```python
from build123d import *

# Parameters (mm, degrees)
F1_DEPTH = 25.4


with BuildPart() as f1:
    # F0 (on Front) → F1 (new body)
    with BuildSketch(Plane.XZ):
        with BuildLine():
            Line((-514.35, 714.375), (-522.739805, 714.375))
            ThreePointArc((-522.739805, 714.375), (-538.640068, 709.542625), (-549.162481, 696.679926))
            Line((-549.162481, 696.679926), (-578.52656, 625.367164))
            ThreePointArc((-578.52656, 625.367164), (-585.141661, 603.436284), (-587.375, 580.638581))
            Line((-587.375, 580.638581), (-587.375, 577.85))
            Line((-587.375, 577.85), (-587.375, 133.35))
            Line((-587.375, 133.35), (-587.375, 130.561419))
            ThreePointArc((-587.375, 130.561419), (-585.141661, 107.763716), (-578.52656, 85.832836))
            Line((-578.52656, 85.832836), (-549.162481, 14.520074))
            ThreePointArc((-549.162481, 14.520074), (-538.640068, 1.657375), (-522.739805, -3.175))
            Line((-522.739805, -3.175), (-514.35, -3.175))
            Line((-514.35, -3.175), (-69.85, -3.175))
            Line((-69.85, -3.175), (-61.460195, -3.175))
            ThreePointArc((-61.460195, -3.175), (-45.559932, 1.657375), (-35.037519, 14.520074))
            Line((-35.037519, 14.520074), (-5.67344, 85.832836))
            ThreePointArc((-5.67344, 85.832836), (0.941661, 107.763716), (3.175, 130.561419))
            Line((3.175, 130.561419), (3.175, 133.35))
            Line((3.175, 133.35), (3.175, 577.85))
            Line((3.175, 577.85), (3.175, 580.638581))
            ThreePointArc((3.175, 580.638581), (0.941661, 603.436284), (-5.67344, 625.367164))
            Line((-5.67344, 625.367164), (-35.037519, 696.679926))
            ThreePointArc((-35.037519, 696.679926), (-45.559932, 709.542625), (-61.460195, 714.375))
            Line((-61.460195, 714.375), (-69.85, 714.375))
            Line((-69.85, 714.375), (-514.35, 714.375))
        make_face()
        with BuildLine():
            Line((-522.739805, 711.2), (-514.35, 711.2))
            Line((-514.35, 711.2), (-69.85, 711.2))
            Line((-69.85, 711.2), (-61.460195, 711.2))
            ThreePointArc((-61.460195, 711.2), (-47.326628, 706.904556), (-37.973371, 695.471045))
            Line((-37.973371, 695.471045), (-8.609293, 624.158284))
            ThreePointArc((-8.609293, 624.158284), (-2.172979, 602.82013), (0, 580.638581))
            Line((0, 580.638581), (0, 577.85))
            Line((0, 577.85), (0, 133.35))
            Line((0, 133.35), (0, 130.561419))
            ThreePointArc((0, 130.561419), (-2.172979, 108.37987), (-8.609293, 87.041716))
            Line((-8.609293, 87.041716), (-37.973371, 15.728955))
            ThreePointArc((-37.973371, 15.728955), (-47.326628, 4.295444), (-61.460195, 0))
            Line((-61.460195, 0), (-69.85, 0))
            Line((-69.85, 0), (-514.35, 0))
            Line((-514.35, 0), (-522.739805, 0))
            ThreePointArc((-522.739805, 0), (-536.873372, 4.295444), (-546.226629, 15.728955))
            Line((-546.226629, 15.728955), (-575.590707, 87.041716))
            ThreePointArc((-575.590707, 87.041716), (-582.027021, 108.37987), (-584.2, 130.561419))
            Line((-584.2, 130.561419), (-584.2, 133.35))
            Line((-584.2, 133.35), (-584.2, 577.85))
            Line((-584.2, 577.85), (-584.2, 580.638581))
            ThreePointArc((-584.2, 580.638581), (-582.027021, 602.82013), (-575.590707, 624.158284))
            Line((-575.590707, 624.158284), (-546.226629, 695.471045))
            ThreePointArc((-546.226629, 695.471045), (-536.873372, 706.904556), (-522.739805, 711.2))
        make_face(mode=Mode.SUBTRACT)
    extrude(amount=F1_DEPTH)


solid = f1.part
```
Work out the finished part from the listing and answer in its coordinate system (mm). A direction names the side the tool comes from. Round coordinates to 2 decimals unless told otherwise and drop trailing zeros. Write each loop counter-clockwise with the first axis right and the second up, starting at its lowest first coordinate (ties: lowest second). Pieces come first, ordered by that corner, then holes. Notation, with made-up numbers: (-17, -37) -> (32, -37) arc R25 ccw to (32, -10) -> close; hole circle Ø4 at (-4.5, 39.25). An arc over 180 degrees is marked (long way). Write each question's results on one line, items separated by ' | '.
Q1. Section B-B, the plane z = 355 is taken. Write down the section's boundary in (x, y) (3 decimals).
Data:
outline: (-587.375, -25.4) -> (-584.2, -25.4) -> (-584.2, 0) -> (-587.375, 0) -> close; (0, -25.4) -> (3.175, -25.4) -> (3.175, 0) -> (0, 0) -> close
Q2. Which of the six approach directions +Z, -Z, +X, -X, +Y, -Y give full straight-line access (tool end or side, diameter ignored) to faces 5 (the flat face through (-23.497, -12.522, 660.314)), 6 (the flat face through (-587.375, -13, 359))?
Data:
face 5: +Y, -Y | face 6: +Z, -Z, -X, +Y, -Y
Q3. Section A-A, the plane x = -295 is taken. Write down the section's boundary in (y, z) (3 decimals).
Data:
outline: (-25.4, -3.175) -> (0, -3.175) -> (0, 0) -> (-25.4, 0) -> close; (-25.4, 711.2) -> (0, 711.2) -> (0, 714.375) -> (-25.4, 714.375) -> close
Q4. Straight lines are drawn through the part: line 1 along Z through (x, y) = (-205, -22.75) (3 decimals); line 2 along X through (y, z) = (-10.5, 560.5) (3 decimals); line 3 along X through (y, z) = (-16.75, 70). For each, find the intervals that lie inside material, in ascending order. Write a range as [from, to].
Data:
line 1: [-3.175, 0], [711.2, 714.375] | line 2: [-587.375, -584.2], [0, 3.175] | line 3: [-572.01, -568.57], [-15.63, -12.19]
Q5. Determine the mould class of faces 1 (the flat face through (-289, -13, 714.375)), 2 (the cylindrical face through (-538.836, -12.522, 1.79)), 3 (the cylindrical face through (-2.113, -12.522, 108.687)), 4 (the flat face through (-20.15, -12.52, 660.52)) for opening direction X: released by +X, released by -X, zero draft, split by the parting line, or undercut.
Data:
face 1: zero draft | face 2: released by -X | face 3: undercut | face 4: released by +X
